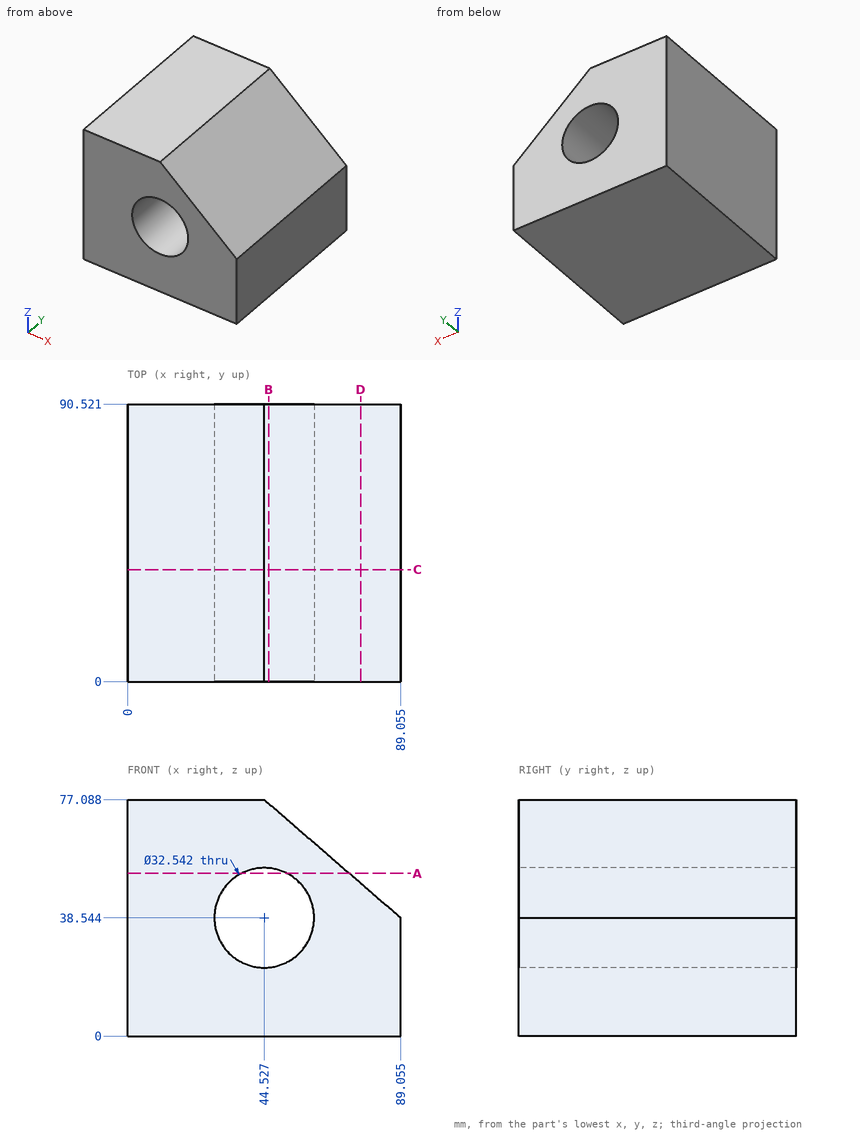
Geometry check sheet. Reference: drawing and pictorial views, mm from the part's lowest x, y, z. Give positions to 0.01 mm unless a question says otherwise; leave off trailing zeros. Order: outer loops, then holes, each group sorted by start corner. A loop starts at its lowest first (then second) coordinate and runs counter-clockwise, first axis right, second up. Notation, with made-up numbers: (23.25, 84) -> (49.25, 84) arc R24 cw to (49.25, 116) -> close; hole circle Ø9 at (-1.5, 7). An arc over 180 degrees is marked (long way). Use CSV: the item, a comma, the result in double quotes. Start each with the question number.
1) Sectioned sample at C-C, the plane y = 36.5. Record the boundary of the cut face in (x, z) (1 decimal).
2) Sectioned sample at D-D, the plane x = 76. Record the boundary of the cut face in (y, z) (1 decimal), plus the area to 3 significant figures.
3) Sectioned sample at B-B, the plane x = 46. Record the boundary of the cut face in (y, z).
4) Material ranges on line 1 (X direction, y = 4.5, z = 53.5) (1 decimal); line 2 (X direction, y = 15, z = 51) (1 decimal); line 3 (Z direction, x = 51, y = 70.5) (1 decimal), recorded low to high. Write a range as from..to.
5) Sectioned sample at A-A, the plane z = 53. Record the boundary of the cut face in (x, y) (1 decimal).
Recorded:
1,outline,"(0, 0) -> (89.1, 0) -> (89.1, 38.5) -> (44.5, 77.1) -> (0, 77.1) -> close; hole circle Ø32.5 at (44.5, 38.5)"
2,outline,"(0, 0) -> (90.5, 0) -> (90.5, 49.8) -> (0, 49.8) -> close"
2,area,"4,510 mm2"
3,outline,"(0, 0) -> (90.52, 0) -> (90.52, 22.34) -> (0, 22.34) -> close; (0, 54.75) -> (90.52, 54.75) -> (90.52, 75.81) -> (0, 75.81) -> close"
4,line 1,"0..38.1, 50.9..71.8"
4,line 2,"0..34.1, 55..74.7"
4,line 3,"0..23.6, 53.5..71.5"
5,outline,"(0, 0) -> (37.1, 0) -> (37.1, 90.5) -> (0, 90.5) -> close; (52, 0) -> (72.4, 0) -> (72.4, 90.5) -> (52, 90.5) -> close"
